```python
from build123d import *

# Parameters (mm, degrees)
SKETCH2_W          = 74.9
SKETCH2_H          = 74.9
BASE_DEPTH         = 7.5
SKETCH3_W          = 40.2
SKETCH3_H          = 40.2
SLOT_DEPTH         = 1.6
CUT_EXTRUDE2_DEPTH = 5.9
FILLET1_R          = 30


with BuildPart() as part:
    # Sketch2 → Base (new body)
    with BuildSketch(Plane(origin=(0, 0, 0), x_dir=(1, 0, 0), z_dir=(0, 1, 0))):
        Rectangle(SKETCH2_W, SKETCH2_H)
    extrude(amount=BASE_DEPTH)

    # Sketch3 → Slot (cut)
    with BuildSketch(Plane(origin=(0, 7.5, 0), x_dir=(1, 0, 0), z_dir=(0, 1, 0))):
        Rectangle(SKETCH3_W, SKETCH3_H)
    extrude(amount=-SLOT_DEPTH, mode=Mode.SUBTRACT)

    # Sketch4 → Cut-Extrude2 (cut)
    with BuildSketch(Plane(origin=(0, 5.9, 0), x_dir=(1, 0, 0), z_dir=(0, 1, 0))):
        Polygon((-19.336485636, -20.1), (-19.336485636, 20.1), (16.190707478, 20.1), (20.1, 16.190707478), (20.1, -16.190707478), (16.190707478, -20.1), align=None)
    extrude(amount=-CUT_EXTRUDE2_DEPTH, mode=Mode.SUBTRACT)

    # Fillet1
    fillet1_edges = [part.edges().sort_by_distance(p)[0] for p in [
        (37.45, 3.75, 37.45),
        (-37.45, 3.75, 37.45),
        (-37.45, 3.75, -37.45),
        (37.45, 3.75, -37.45),
    ]]
    fillet(fillet1_edges, radius=FILLET1_R)


solid = part.part
```
Design review of the part built by this model. Coordinates are the model's own, in mm. A direction names the side the tool comes from. Round coordinates to 2 decimals unless told otherwise and drop trailing zeros. Order: outer loops, then holes, each group sorted by start corner. A loop starts at its lowest first (then second) coordinate and runs counter-clockwise, first axis right, second up. Notation, with made-up numbers: (11.5, 13) - (29.5, 13) arc R16 cw to (29.5, 37) - close; hole circle Ø8 at (10.5, 6). An arc over 180 degrees is marked (long way). Return JSON: item names as keys, results as strings.
Q1. Consider section D-D on x = -17. Write out the cut boundary in (y, z), plus the area to 3 significant figures.
Computed values:
{"outline": "(0, -35.89) - (7.5, -35.89) - (7.5, -20.1) - (0, -20.1) - close; (0, 20.1) - (7.5, 20.1) - (7.5, 35.89) - (0, 35.89) - close", "area": "237 mm2"}
Q2. Consider section A-A on x = -0.5. Write out the cut boundary in (y, z), plus the area to 3 significant figures.
Computed values:
{"outline": "(0, -37.45) - (7.5, -37.45) - (7.5, -20.1) - (0, -20.1) - close; (0, 20.1) - (7.5, 20.1) - (7.5, 37.45) - (0, 37.45) - close", "area": "260 mm2"}
Q3. Wall thickness on L1, parallel to Z at x = 8.5, y = 5; L2, parallel to X at y = 7.25, z = 3; L3, parallel to X at y = 3.75, z = -6.5: over which ranges is each line inside the solid? List them lowest first. Write a range as [from, to].
Computed values:
{"L1": "z = [-37.43, -20.1], [20.1, 37.43]", "L2": "x = [-37.45, -20.1], [20.1, 37.45]", "L3": "x = [-37.45, -19.34], [20.1, 37.45]"}
Q4. Machinability: for faces 4 (the flat face through (19, 5.9, -19)), 5 (the flat face through (0, 4, 37.45)), 6 (the flat face through (18.17, 2.99, 18.12)), which of the approach directions +Z, -Z, +X, -X, +Y, -Y give a long, thin tool a straight path to every point of the face, cutting with its end or side? Answer none if there is none.
Computed values:
{"face 4": "+Y", "face 5": "+Z, +X, -X, +Y, -Y", "face 6": "+Y, -Y"}
Q5. For pin 1 Ø1.5 at (x, y) = (28.5, 3) entering from +Z; pin 2 Ø3 at (x, z) = (17.5, 18.5) entering from +Y, all flat-tipped, find the tip position at first contact; note any pin that passes through.
Computed values:
{"pin 1": "stops at z = 29.54", "pin 2": "stops at y = 5.9"}
Q6. Consider section B-B on y = 3.25. Write out the cut boundary in (x, z).
Computed values:
{"outline": "(-37.45, -7.45) arc R30 ccw to (-7.45, -37.45) - (7.45, -37.45) arc R30 ccw to (37.45, -7.45) - (37.45, 7.45) arc R30 ccw to (7.45, 37.45) - (-7.45, 37.45) arc R30 ccw to (-37.45, 7.45) - close; hole (-19.34, -20.1) - (16.19, -20.1) - (20.1, -16.19) - (20.1, 16.19) - (16.19, 20.1) - (-19.34, 20.1) - close"}
Q7. The part is to be moulded in two halves that separate along X. For faces 1 (the flat face through (-20.1, 7, 0)), 2 (the flat face through (37.45, 4, 0)), 3 (the flat face through (-37.45, 4, 0)), say which applies: pulls with the +X half, pulls with the -X half, needs draft (parallel to the pull), parting line crosses it, or undercut.
Computed values:
{"face 1": "undercut", "face 2": "pulls with the +X half", "face 3": "pulls with the -X half"}
Q8. Consider section C-C on z = -4. Write out the cut boundary in (x, y), plus the area to 3 significant figures.
Computed values:
{"outline": "(-37.45, 0) - (-19.34, 0) - (-19.34, 5.9) - (-20.1, 5.9) - (-20.1, 7.5) - (-37.45, 7.5) - close; (20.1, 0) - (37.45, 0) - (37.45, 7.5) - (20.1, 7.5) - close", "area": "265 mm2"}
